Drawing for the job (mm, zero at the part's lowest x, y, z). Give positions to 0.01 mm unless a question says otherwise; leave off trailing zeros. Order: outer loops, then holes, each group sorted by start corner. A loop starts at its lowest first (then second) coordinate and runs counter-clockwise, first axis right, second up. Notation, with made-up numbers: (7.5, 88) -> (27.5, 88) arc R25 cw to (27.5, 117) -> close; hole circle Ø8 at (31, -0.5). An arc over 180 degrees is marked (long way). Use a Markdown table: item, result. Add a question column.
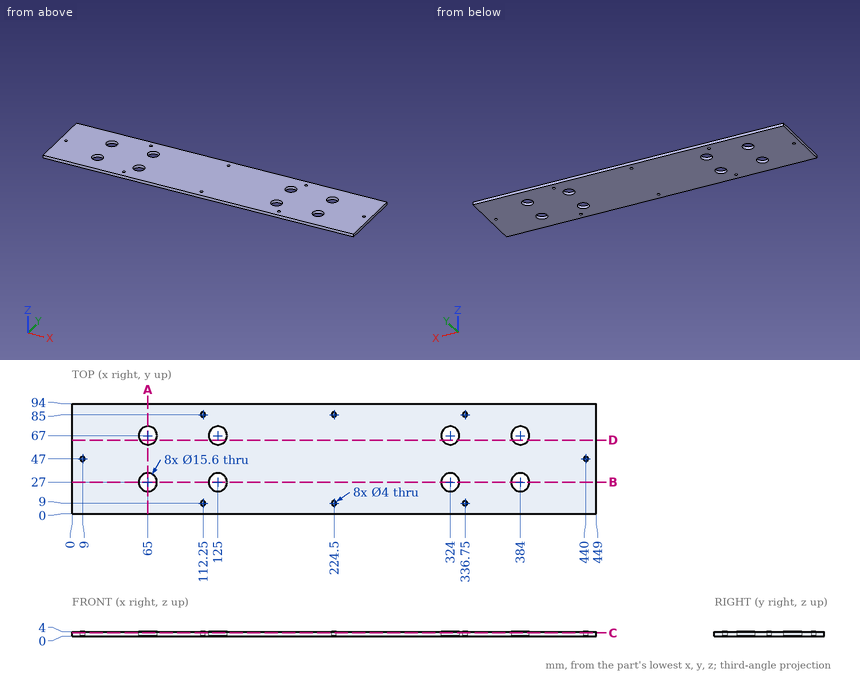
(1) Band-saw the part on C-C on z = 2.95. State how many separate pieces and enclosed holes the cut face has, plus the area to 3 significant figures.
(2) Pin check, flat tips, straight feed: pin 1 Ø12.5 at (x, y) = (65, 27) entering from -Z; pin 2 Ø1 at (y, z) = (42, 0.5) entering from -X. Stop position of each tip, or through.
(3) Band-saw the part on D-D on y = 63. Give the cut face in (x, z).
(4) Band-saw the part on A-A on x = 65. Give the cut face in (y, z), plus the area to 3 significant figures.
(5) Wall check: probe 1 along Y at (x, z) = (224.5, 2.7); probe 2 along Y at (x, z) = (65, 2.45); probe 3 along X at (y, z) = (28, 1.1). Give the ranges that are in metal, low to high.
(6) Band-saw the part on B-B on y = 27. Give the cut face in (x, z).
Response:
| question | item | result |
|---|---|---|
| 1 | separate pieces | 1 |
| 1 | enclosed holes | 16 |
| 1 | area | 40,600 mm² |
| 2 | pin 1 | passes through |
| 2 | pin 2 | stops at x = 0 |
| 3 | outline | (0, 0) -> (58.3, 0) -> (58.3, 4) -> (0, 4) -> close; (71.7, 0) -> (118.3, 0) -> (118.3, 4) -> (71.7, 4) -> close; (131.7, 0) -> (317.3, 0) -> (317.3, 4) -> (131.7, 4) -> close; (330.7, 0) -> (377.3, 0) -> (377.3, 4) -> (330.7, 4) -> close; (390.7, 0) -> (449, 0) -> (449, 4) -> (390.7, 4) -> close |
| 4 | outline | (0, 0) -> (19.2, 0) -> (19.2, 4) -> (0, 4) -> close; (34.8, 0) -> (59.2, 0) -> (59.2, 4) -> (34.8, 4) -> close; (74.8, 0) -> (94, 0) -> (94, 4) -> (74.8, 4) -> close |
| 4 | area | 251 mm² |
| 5 | probe 1 | y = 0 to 7, 11 to 83, 87 to 94 |
| 5 | probe 2 | y = 0 to 19.2, 34.8 to 59.2, 74.8 to 94 |
| 5 | probe 3 | x = 0 to 57.26, 72.74 to 117.26, 132.74 to 316.26, 331.74 to 376.26, 391.74 to 449 |
| 6 | outline | (0, 0) -> (57.2, 0) -> (57.2, 4) -> (0, 4) -> close; (72.8, 0) -> (117.2, 0) -> (117.2, 4) -> (72.8, 4) -> close; (132.8, 0) -> (316.2, 0) -> (316.2, 4) -> (132.8, 4) -> close; (331.8, 0) -> (376.2, 0) -> (376.2, 4) -> (331.8, 4) -> close; (391.8, 0) -> (449, 0) -> (449, 4) -> (391.8, 4) -> close |
